Geometry: final body of the model. Coordinates: model frame, mm. Coordinates: 2 decimals unless noted, no trailing zeros. Order: outer loops, then holes, each group sorted by start corner. A loop starts at its lowest first (then second) coordinate and runs counter-clockwise, first axis right, second up. Notation, with made-up numbers: (-12, 44) - (-4, 44) arc R22 cw to (-4, 56) - close; hole circle Ø8 at (79.25, 83.5). An arc over 180 degrees is marked (long way). Use a Markdown table: item, result. Add a question column.
Autodesk Inventor part; units mm, degrees
ref_plane "YZ Plane" through (0, 0, 0) normal (1, 0, 0) x (0, 1, 0)
ref_plane "XZ Plane" through (0, 0, 0) normal (0, 1, 0) x (-1, 0, 0)
ref_plane "XY Plane" through (0, 0, 0) normal (0, 0, 1) x (1, 0, 0)
ref_plane "Work Plane1" through (0, 0, 0) normal (0, 0, 1) x (1, 0, 0)
sketch "Sketch1" plane through (0, 0, 0) normal (0, 0, 1) x (1, 0, 0)
  circle A0 centre (-12.1, 23.75) radius 2.15 construction
  circle A1 centre (13.2, 23.75) radius 2.15 construction
  circle A2 centre (-12.1, 31.75) radius 2.15 construction
  circle A3 centre (13.2, 31.75) radius 2.15 construction
  line L0 (-12.1, 23.75) -> (13.2, 23.75) construction
  line L1 (-12.1, 21.25) -> (13.2, 21.25)
  line L2 (13.2, 26.25) -> (-12.1, 26.25)
  arc A4 (-12.1, 26.25) -> (-12.1, 21.25) centre (-12.1, 23.75) ccw
  arc A5 (13.2, 21.25) -> (13.2, 26.25) centre (13.2, 23.75) ccw
  point P0 (0, 0)
  point P1 (0.55, 23.75)
  dimension "d0" = 5
extrude "Extrusion1" add sketch "Sketch1" along normal blind 5
sketch "Sketch2" plane through (0, 0, 5) normal (0, 0, 1) x (1, 0, 0)
  arc A0 (13.2, 21.25) -> (13.2, 26.25) centre (13.2, 23.75) ccw construction
  line L0 (13.2, 26.25) -> (-12.1, 26.25) construction
  arc A1 (-12.1, 26.25) -> (-12.1, 21.25) centre (-12.1, 23.75) ccw construction
  line L1 (-12.1, 21.25) -> (13.2, 21.25) construction
  point P0 (0, 0)
hole "Hole1" at (13.2, 23.75, 5) at (-12.1, 23.75, 5) direction (0, 0, -1) diameter 3.4 depth 7
properties part number "TinyBeltClamp"
1) Section A-A (z = 0.8). Return loops of the section in (x, y).
2) Ray query, line 1 along X through (y, z) = (23.9, 3); line 2 along Y through (x, z) = (13.2, 3). Return the intervals inside material, ascending.
3) Draft query along Y for faces 1 (the face through (0, 21.25, 2)), 2 (the face through (13.9, 22.2, 2.5)), 3 (the face through (-10.59, 22.97, 2.46)), 4 (the face through (15.7, 23.8, 2.5)). Return one class per face: pulls with the +Y half, pulls with the -Y half, needs draft (parallel to the pull), parting line crosses it, or undercut.
4) Pin query (flat end, axial travel): pin 1 (3 mm diameter, centred on x = 13.2, y = 23.75, fed in from -Z). Return the tip coordinate at first contact, or that it passes through.
5) Section B-B (y = 23.75). Return loops of the section in (x, z), then the cut area to 4 significant figures.
Values follow:
| question | item | result |
|---|---|---|
| 1 | outline | (-12.1, 21.25) - (13.2, 21.25) arc R2.5 ccw to (13.2, 26.25) - (-12.1, 26.25) arc R2.5 ccw to start; hole circle Ø3.4 at (-12.1, 23.75); hole circle Ø3.4 at (13.2, 23.75) |
| 2 | line 1 | x = -14.6 to -13.79, -10.41 to 11.51, 14.89 to 15.7 |
| 2 | line 2 | y = 21.25 to 22.05, 25.45 to 26.25 |
| 3 | face 1 | pulls with the -Y half |
| 3 | face 2 | undercut |
| 3 | face 3 | undercut |
| 3 | face 4 | parting line crosses it |
| 4 | pin 1 | passes through |
| 5 | outline | (-14.6, 0) - (-13.8, 0) - (-13.8, 5) - (-14.6, 5) - close; (-10.4, 0) - (11.5, 0) - (11.5, 5) - (-10.4, 5) - close; (14.9, 0) - (15.7, 0) - (15.7, 5) - (14.9, 5) - close |
| 5 | area | 117.5 mm² |
